```python
from build123d import *

# Parameters (mm, degrees)
SKETCH1_W           = 10
SKETCH1_H           = 7
BOSS_EXTRUDE1_DEPTH = 6
SKETCH4_R           = 1.25
CUT_EXTRUDE1_DEPTH  = 6
FILLET1_R           = 1


with BuildPart() as part:
    # Sketch1 → Boss-Extrude1 (new body)
    with BuildSketch(Plane.XY):
        Rectangle(SKETCH1_W, SKETCH1_H)
    extrude(amount=BOSS_EXTRUDE1_DEPTH)

    # Sketch3 → Cut-Loft2 section 0
    with BuildSketch(Plane(origin=(0, 0, 0), x_dir=(-1, 0, 0), z_dir=(0, 0, -1))):
        with BuildLine():
            Line((-3.306604223, -2.5), (-0.806604223, -2.5))
            Line((-0.806604223, -2.5), (-0.806604223, 2.5))
            Line((-0.806604223, 2.5), (-3.306604223, 2.5))
            Line((-3.306604223, 2.5), (-3.306604223, -2.5))
        make_face()
    # Sketch2 → Cut-Loft2 section 1
    with BuildSketch(Plane.XY.offset(6)):
        with BuildLine():
            Line((0.806604223, -3), (3.306604223, -3))
            Line((3.306604223, -3), (3.306604223, 3))
            Line((3.306604223, 3), (0.806604223, 3))
            Line((0.806604223, 3), (0.806604223, -3))
        make_face()
    loft(mode=Mode.SUBTRACT)

    # Sketch4 → Cut-Extrude1 (cut)
    with BuildSketch(Plane.XY.offset(6)):
        with Locations((-2.858867823, 0)):
            Circle(SKETCH4_R)
    extrude(amount=-CUT_EXTRUDE1_DEPTH, mode=Mode.SUBTRACT)

    # Fillet1
    # the kernel refuses this fillet: 1 mm, written as the material it takes off along each edge
    with BuildSketch(Plane(origin=(-7.5, -3.5, 0), x_dir=(0, 0, 1), z_dir=(1, 0, 0)), Plane(origin=(7.5, 3.5, 6), x_dir=(0, -1, 0), z_dir=(-1, 0, 0))) as fillet1_piece_1:
        with BuildLine():
            CenterArc((FILLET1_R, -FILLET1_R), FILLET1_R, 90, 90)
            Line((0, -FILLET1_R), (0, 0))
            Line((0, 0), (FILLET1_R, 0))
        make_face()
    extrude(amount=15, mode=Mode.SUBTRACT)
    with BuildSketch(Plane(origin=(7.5, 3.5, 0), x_dir=(0, -1, 0), z_dir=(-1, 0, 0)), Plane(origin=(-7.5, -3.5, 6), x_dir=(0, 0, -1), z_dir=(1, 0, 0))) as fillet1_piece_2:
        with BuildLine():
            CenterArc((FILLET1_R, FILLET1_R), FILLET1_R, 180, 90)
            Line((0, FILLET1_R), (0, 0))
            Line((0, 0), (FILLET1_R, 0))
        make_face()
    extrude(amount=15, mode=Mode.SUBTRACT)
    with BuildSketch(Plane(origin=(-5, -3.5, -2.5), x_dir=(1, 0, 0), z_dir=(0, 0, 1)), Plane(origin=(-5, 3.5, -2.5), x_dir=(0, -1, 0), z_dir=(0, 0, 1))) as fillet1_piece_3:
        with BuildLine():
            CenterArc((FILLET1_R, FILLET1_R), FILLET1_R, 180, 90)
            Line((0, FILLET1_R), (0, 0))
            Line((0, 0), (FILLET1_R, 0))
        make_face()
    extrude(amount=11, mode=Mode.SUBTRACT)
    with BuildSketch(Plane(origin=(5, -3.5, -2.5), x_dir=(-1, 0, 0), z_dir=(0, 0, 1)), Plane(origin=(5, 3.5, -2.5), x_dir=(0, -1, 0), z_dir=(0, 0, 1))) as fillet1_piece_4:
        with BuildLine():
            CenterArc((FILLET1_R, -FILLET1_R), FILLET1_R, 90, 90)
            Line((0, -FILLET1_R), (0, 0))
            Line((0, 0), (FILLET1_R, 0))
        make_face()
    extrude(amount=11, mode=Mode.SUBTRACT)


solid = part.part
```
CAD build for the part. Positions are in the model's coordinates, mm. A direction names the side the tool comes from. Coordinates: 2 decimals unless noted, no trailing zeros. Order: outer loops, then holes, each group sorted by start corner. A loop starts at its lowest first (then second) coordinate and runs counter-clockwise, first axis right, second up. Notation, with made-up numbers: (20.5, -31) - (77.5, -31) arc R20 ccw to (77.5, 2) - close; hole circle Ø10 at (73, 80.25). An arc over 180 degrees is marked (long way). Answer in a Markdown table with one row per item.
1. Slice it at B-B, the plane y = 0. Give the number of separate pieces and of enclosed holes in the cut face, then the cut area to 3 significant figures.
Answer:
| item | result |
|---|---|
| separate pieces | 3 |
| enclosed holes | 0 |
| area | 30.0 mm² |
2. Drill centre lines: L1, parallel to X at y = 0.75, z = 2.75; L2, parallel to X at y = 2.25, z = 1; L3, parallel to X at y = 1, z = 0.5. Where is each one in solid material? Low to high. Write a range as from..to.
Answer:
| item | result |
|---|---|
| L1 | -5..-3.86, -1.86..0.81, 3.31..5 |
| L2 | -5..0.81, 3.31..5 |
| L3 | -5..-3.61, -2.11..0.81, 3.31..5 |
3. Flat gauge pin, fed straight in: P1, Ø1.5, axis at x = -2.86, y = 0, coming from the -Z side (1 decimal). Where does the tip first touch, or does it go through?
Answer:
| item | result |
|---|---|
| P1 | through |
4. 3-axis set-ups, long thin cutter, end or side, ignore diameter. For faces 4 (the face through (2.07, -2.75, 2.98)), 5 (the face through (-4.699, 3.215, 2.958)): which of +Z, -Z, +X, -X, +Y, -Y reach the whole face in a straight line?
Answer:
| item | result |
|---|---|
| face 4 | +Z |
| face 5 | +Z, -Z, -X, +Y |
5. Pull direction Y, two halves, no side cores. Call faces 1 (the face through (2.04, 2.75, 2.98)), 2 (the face through (-1, 0, 6)), 3 (the face through (0.07, 3.199, 5.715)): +Y half, -Y half, draft (parallel to the pull), parting line (faces both ways), or undercut.
Answer:
| item | result |
|---|---|
| face 1 | undercut |
| face 2 | draft |
| face 3 | +Y half |
6. Slice it at A-A, the plane x = 3.75. List the corners of the cut face in (y, z).
Answer:
| item | result |
|---|---|
| outline | (-3.5, 1) arc R1 ccw to (-2.5, 0) - (2.5, 0) arc R1 ccw to (3.5, 1) - (3.5, 5) arc R1 ccw to (2.5, 6) - (-2.5, 6) arc R1 ccw to (-3.5, 5) - close |
